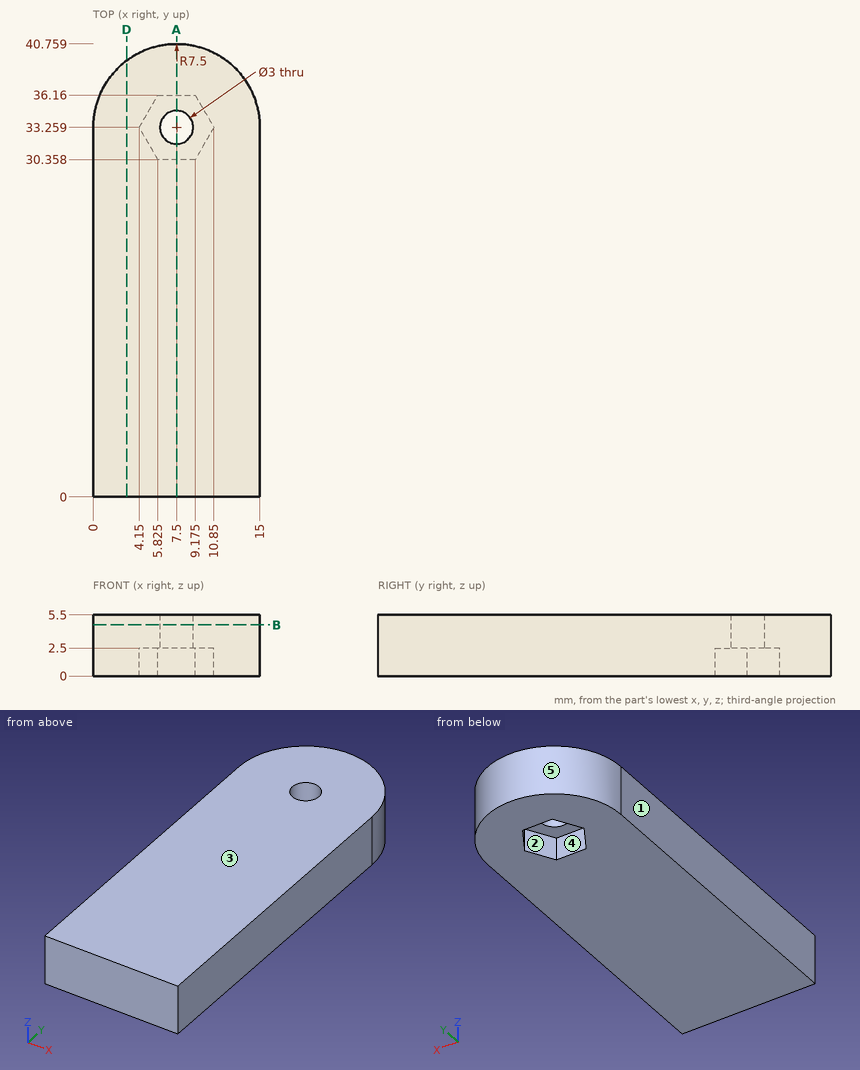
Study the drawing (mm; zero at the part's minimum x, y, z) and answer. A direction names the side the tool comes from. Coordinates: 2 decimals unless noted, no trailing zeros. Write each loop counter-clockwise with the first axis right and the second up, starting at its lowest first coordinate (ties: lowest second). Pieces come first, ordered by that corner, then holes. Notation, with made-up numbers: (62.5, 77) - (90.5, 77) arc R10 ccw to (90.5, 86) - close; hole circle Ø9 at (-33.5, 13.5). An arc over 180 degrees is marked (long way). Answer as a JSON object with one key per item and string values. Group by question number.
1. A cutting plane is placed at A-A (x = 7.5). Determine the outline of the cut face in (y, z), plus the area to 3 significant figures.
2. Consider L1, parallel to Y at x = 7.5, z = 4.6; L2, parallel to Y at x = 9.5, z = 0.9 (1 decimal); L3, parallel to X at y = 32, z = 5.3 (1 decimal). Determine where each line is inside the solid, lowest interval first. Write a range as [from, to].
3. Each of these flat-tipped pins is pushed along its axis until it touches: P1, Ø1.5, axis at x = 3, z = 1, coming from the +Y side (1 decimal); P2, Ø2.5, axis at x = 7.5, y = 33.26, coming from the +Z side; P3, Ø1, axis at x = 3, z = 0.5, coming from the +Y side. Where does it stop, or does it pass through?
4. Which of the six approach directions +Z, -Z, +X, -X, +Y, -Y give full straight-line access (tool end or side, diameter ignored) to the marked faces 1 and 2?
5. A cutting plane is placed at B-B (z = 4.6). Determine the outline of the cut face in (x, y), plus the area to 3 significant figures.
6. A cutting plane is placed at D-D (x = 3). Determine the outline of the cut face in (y, z).
7. The mould has two halves that part along Y. Classify the marked faces 3, 4 and 5: +Y half, -Y half, draft (parallel to the pull), parting line (faces both ways), or undercut.
Worked out:
{
 "1": {"outline": "(0, 0) - (30.36, 0) - (30.36, 2.5) - (31.76, 2.5) - (31.76, 5.5) - (0, 5.5) - close; (34.76, 2.5) - (36.16, 2.5) - (36.16, 0) - (40.76, 0) - (40.76, 5.5) - (34.76, 5.5) - close", "area": "201 mm²"},
 "2": {"L1": "y = [0, 31.76], [34.76, 40.76]", "L2": "y = [0, 30.9], [35.6, 40.5]", "L3": "x = [0, 6.7], [8.3, 15]"},
 "3": {"P1": "stops at y = 39.8", "P2": "passes through", "P3": "stops at y = 39.6"},
 "4": {"face 1": "+Z, -Z, -X, +Y, -Y", "face 2": "-Z"},
 "5": {"outline": "(0, 0) - (15, 0) - (15, 33.26) arc R7.5 ccw to (0, 33.26) - close; hole circle Ø3 at (7.5, 33.26)", "area": "580 mm²"},
 "6": {"outline": "(0, 0) - (39.26, 0) - (39.26, 5.5) - (0, 5.5) - close"},
 "7": {"face 3": "draft", "face 4": "undercut", "face 5": "+Y half"}
}
